Work out the finished part from the listing and answer in its coordinate system (mm). Face numbers are marked on the shaded views. A direction names the side the tool comes from. Coordinates: 2 decimals unless noted, no trailing zeros. Loops run counter-clockwise (first coordinate to the right, second up) from the corner with the lowest first, then second, coordinate; pieces in that order, holes last. Notation, with made-up numbers: (73, 79) - (123, 79) arc R22 ccw to (123, 90) - close; hole circle Ø5 at (-9, 42). An arc over 180 degrees is marked (long way). Write each question's results on one line, items separated by ' | '. Start each with the question number.
Item 1: Section A-A, the plane y = 0 is taken. Write down the section's boundary in (x, z), plus the area to 3 significant figures.
Item 2: A tool of negligible diameter and unlimited length cuts with its end or side. For the marked faces 1 and 2, from which of +Z, -Z, +X, -X, +Y, -Y can it reach the whole face along a straight path? Write none if from no direction.
Item 3: Consider probe 1 along Y at (x, z) = (-18, -1.25); probe 2 along X at (y, z) = (16, 2.25); probe 3 along X at (y, z) = (-9, 0). Determine where each line is inside the solid, lowest interval first. Write a range as [from, to].
Item 4: Section C-C, the plane y = 21 is taken. Write down the section's boundary in (x, z).
Item 5: Section D-D, the plane x = -2 is taken. Write down the section's boundary in (y, z), plus the area to 3 significant figures.
Item 6: Each of these flat-tipped pins is pushed along its axis until it touches: pin 1 Ø1 at (x, y) = (26, 21.5) entering from +Z; pin 2 Ø2 at (x, z) = (21.5, 1) entering from +Y; pin 3 Ø1 at (y, z) = (18, -1) entering from +X. Where does it stop, or does it pass through?
Item 7: For a pull along X with two mould halves and no side action, classify the marked faces 3 and 4 as +X half, -X half, draft (parallel to the pull), parting line (faces both ways), or undercut.
Item 8: Section B-B, the plane x = 22.5 is taken. Write down the section's boundary in (y, z).
from build123d import *

# Parameters (mm, degrees)
SKETCH1_R           = 37.5
SKETCH1_W           = 7.071067812
SKETCH1_H           = 7.071067812
BOSS_EXTRUDE1_DEPTH = 2.5
CUT_EXTRUDE1_DEPTH  = 4
CIRPATTERN1_COUNT   = 6
SKETCH4_R           = 8.302662018
SKETCH4_W           = 7.071067812
SKETCH4_H           = 7.071067812
BOSS_EXTRUDE2_DEPTH = 2


with BuildPart() as part:
    # Sketch1 → Boss-Extrude1 (new, symmetric)
    with BuildSketch(Plane.XY):
        Circle(SKETCH1_R)
        Rectangle(SKETCH1_W, SKETCH1_H, mode=Mode.SUBTRACT)
    extrude(amount=BOSS_EXTRUDE1_DEPTH, both=True)

    # Sketch2 → Cut-Extrude1 (cut, symmetric)
    with BuildSketch(Plane.XY):
        with BuildLine():
            Line((0, 9.158641407), (-12.037071564, 26.115211784))
            ThreePointArc((-12.037071564, 26.115211784), (-6.351662121, 29.087034336), (0, 29.988143709))
            ThreePointArc((0, 29.988143709), (6.351662121, 29.087034336), (12.037071564, 26.115211784))
            Line((12.037071564, 26.115211784), (0, 9.158641407))
        make_face()
    cut_extrude1 = extrude(amount=CUT_EXTRUDE1_DEPTH, both=True, mode=Mode.SUBTRACT)

    # CirPattern1: Cut-Extrude1 ×6 about axis
    cirpattern1_axis = Axis((0, 0, 0), (0, 0, 1))
    for i in range(1, CIRPATTERN1_COUNT):
        add(cut_extrude1.rotate(cirpattern1_axis, i * 360 / CIRPATTERN1_COUNT), mode=Mode.SUBTRACT)

    # Sketch4 → Boss-Extrude2 (add)
    with BuildSketch(Plane.XY.offset(2.5)):
        Circle(SKETCH4_R)
        Rectangle(SKETCH4_W, SKETCH4_H, mode=Mode.SUBTRACT)
    extrude(amount=BOSS_EXTRUDE2_DEPTH)


solid = part.part
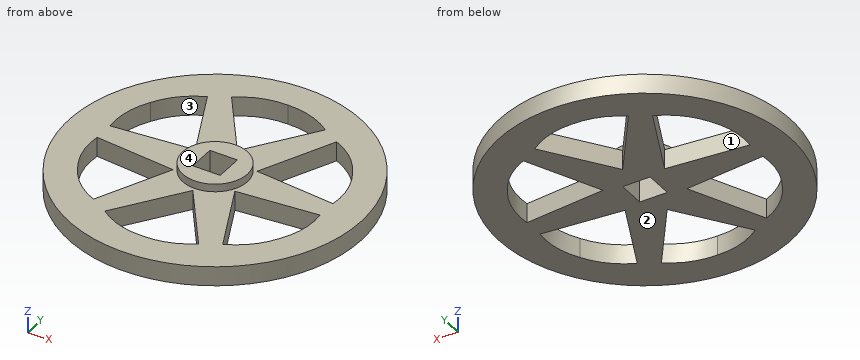
Answer key:
1) outline: (-37.5, -2.5) - (-3.54, -2.5) - (-3.54, 4.5) - (-8.3, 4.5) - (-8.3, 2.5) - (-37.5, 2.5) - close; (3.54, -2.5) - (37.5, -2.5) - (37.5, 2.5) - (8.3, 2.5) - (8.3, 4.5) - (3.54, 4.5) - close | area: 359 mm^2
2) face 1: +Z, -Z | face 2: -Z, +X, -X, +Y, -Y
3) probe 1: y = [-32.9, -22.83], [-3.63, 3.63], [22.83, 32.9] | probe 2: x = [-33.92, -25.39], [-13.17, -4.86], [4.86, 13.17], [25.39, 33.92] | probe 3: x = [-36.4, -28.38], [-9.96, 9.96], [28.38, 36.4]
4) outline: (-31.07, -2.5) - (-20.87, -2.5) - (-20.87, 2.5) - (-31.07, 2.5) - close; (-15.46, -2.5) - (-8.41, -2.5) - (-8.41, 2.5) - (-15.46, 2.5) - close; (8.41, -2.5) - (15.46, -2.5) - (15.46, 2.5) - (8.41, 2.5) - close; (20.87, -2.5) - (31.07, -2.5) - (31.07, 2.5) - (20.87, 2.5) - close
5) outline: (-37.45, -2.5) - (-29.94, -2.5) - (-29.94, 2.5) - (-37.45, 2.5) - close; (-11.98, -2.5) - (-3.54, -2.5) - (-3.54, 4.5) - (-8.06, 4.5) - (-8.06, 2.5) - (-11.98, 2.5) - close; (3.54, -2.5) - (11.98, -2.5) - (11.98, 2.5) - (8.06, 2.5) - (8.06, 4.5) - (3.54, 4.5) - close; (29.94, -2.5) - (37.45, -2.5) - (37.45, 2.5) - (29.94, 2.5) - close | area: 178 mm^2
6) pin 1: stops at z = 2.5 | pin 2: stops at y = 31.4 | pin 3: stops at x = 33.17
7) face 3: undercut | face 4: draft
8) outline: (-30, -2.5) - (-19.59, -2.5) - (-19.59, 2.5) - (-30, 2.5) - close; (-3.21, -2.5) - (3.21, -2.5) - (3.21, 2.5) - (-3.21, 2.5) - close; (19.59, -2.5) - (30, -2.5) - (30, 2.5) - (19.59, 2.5) - close
